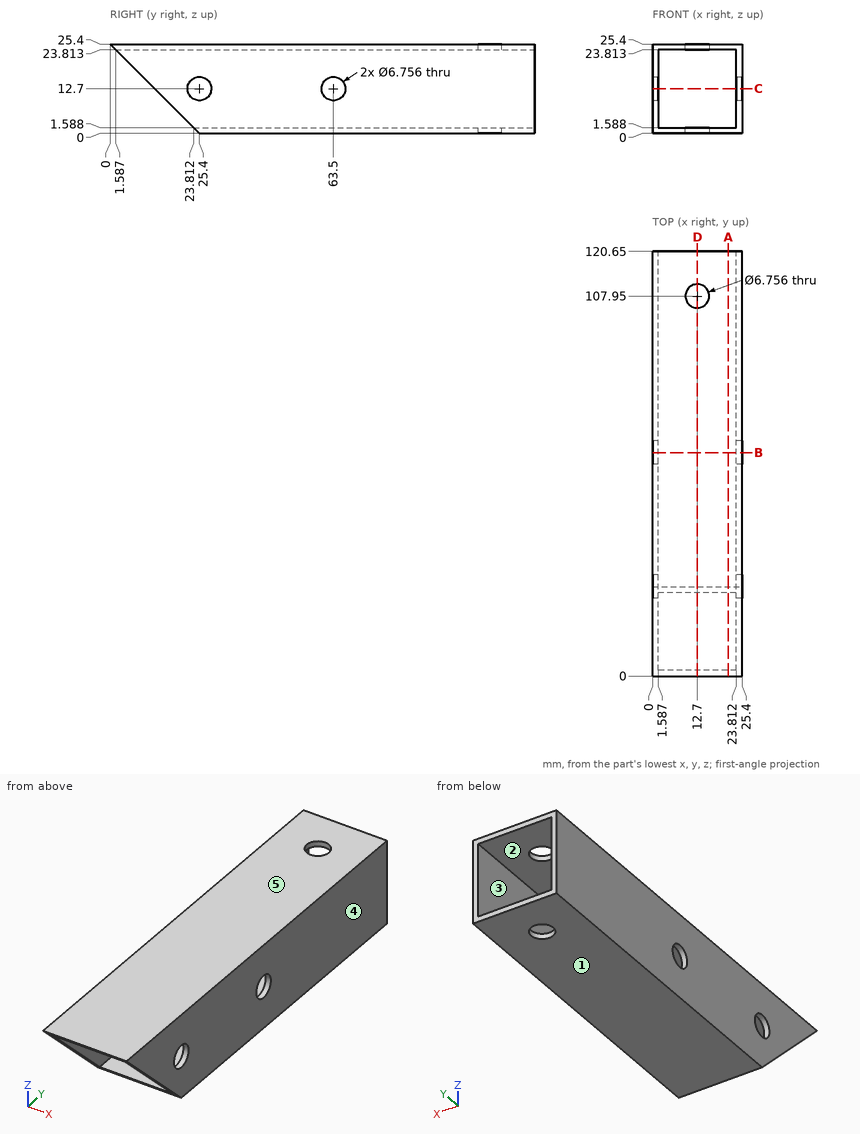
Part print with two shaded views. Sizes in mm from the minimum x, y, z corner. A direction names the side the tool comes from. Round coordinates to 2 decimals unless told otherwise and drop trailing zeros. Loops run counter-clockwise (first coordinate to the right, second up) from the corner with the lowest first, then second, coordinate; pieces in that order, holes last. Notation, with made-up numbers: M 60,14.25 L 108,14.25 A20 ccw 108,43.25 Z; hole C 80,6.25 d9. An arc over 180 degrees is marked long. Put each result on its own line as item: value. Start each with the question number.
Item 1: Drop a flat-ended pin along its axis: P1, Ø2, axis at x = 3, z = 7.5, coming from the +Y side. Give the stop position or say it passes through.
Item 2: 3-axis set-ups, long thin cutter, end or side, ignore diameter. For the marked faces 1 and 2: which of +Z, -Z, +X, -X, +Y, -Y reach the whole face in a straight line?
Item 3: Cut at D-D (x = 12.7). List the corners of the cut face in (y, z).
Item 4: Mould opens along Z. For the marked faces 3, 4 and 5 say: released by +Z, released by -Z, zero draft, split by the parting line, or undercut.
Item 5: Cut at A-A (x = 21.5). List the corners of the cut face in (y, z).
Item 6: Cut at B-B (y = 63.5). List the corners of the cut face in (x, z), then the cut area to 3 significant figures.
Item 7: Cut at C-C (z = 12.7). List the corners of the cut face in (x, y).
Item 8: Drill centre lines: line 1 along Z through (x, y) = (17.5, 67.5); line 2 along Y through (x, z) = (12.7, 0.3). Where is each one in solid material? Low to high.
Answer block:
1. P1: through
2. face 1: -Z, +X, -X, +Y, -Y
2. face 2: +Y, -Y
3. outline: M 0,25.4 L 1.59,23.81 L 104.57,23.81 L 104.57,25.4 Z; M 23.81,1.59 L 25.4,0 L 104.57,0 L 104.57,1.59 Z; M 111.33,0 L 120.65,0 L 120.65,1.59 L 111.33,1.59 Z; M 111.33,23.81 L 120.65,23.81 L 120.65,25.4 L 111.33,25.4 Z
4. face 3: undercut
4. face 4: zero draft
4. face 5: released by +Z
5. outline: M 0,25.4 L 1.59,23.81 L 120.65,23.81 L 120.65,25.4 Z; M 23.81,1.59 L 25.4,0 L 120.65,0 L 120.65,1.59 Z
6. outline: M 0,0 L 25.4,0 L 25.4,9.32 L 23.81,9.32 L 23.81,1.59 L 1.59,1.59 L 1.59,9.32 L 0,9.32 Z; M 0,16.08 L 1.59,16.08 L 1.59,23.81 L 23.81,23.81 L 23.81,16.08 L 25.4,16.08 L 25.4,25.4 L 0,25.4 Z
6. area: 130 mm2
7. outline: M 0,12.7 L 1.59,12.7 L 1.59,22.02 L 0,22.02 Z; M 0,28.78 L 1.59,28.78 L 1.59,60.12 L 0,60.12 Z; M 0,66.88 L 1.59,66.88 L 1.59,120.65 L 0,120.65 Z; M 23.81,12.7 L 25.4,12.7 L 25.4,22.02 L 23.81,22.02 Z; M 23.81,28.78 L 25.4,28.78 L 25.4,60.12 L 23.81,60.12 Z; M 23.81,66.88 L 25.4,66.88 L 25.4,120.65 L 23.81,120.65 Z
8. line 1: 0 to 1.59, 23.81 to 25.4
8. line 2: 25.1 to 104.57, 111.33 to 120.65
